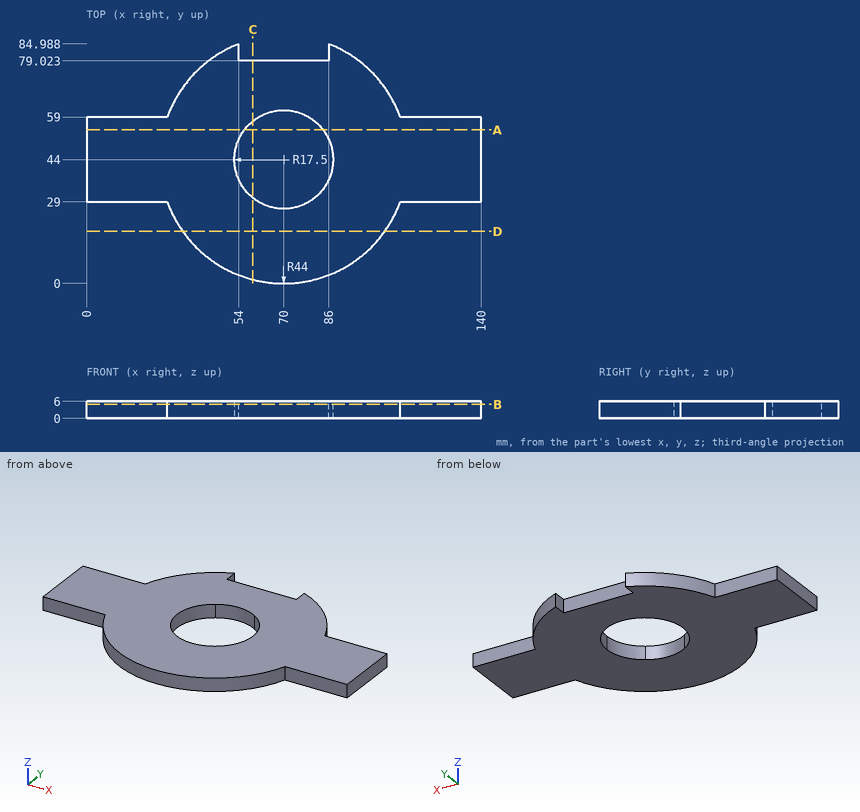
Job drawing, mm, ordinate dimensions from the low corner. One solid piece. Give positions to 0.01 mm unless a question says otherwise; leave off trailing zeros. Write each loop counter-clockwise with the first axis right and the second up, starting at its lowest first coordinate (ties: lowest second). Pieces come first, ordered by that corner, then holes. Notation, with made-up numbers: (-30.75, 5) - (22.25, 5) arc R33 ccw to (22.25, 34) - close; hole circle Ø11 at (76, 8). An arc over 180 degrees is marked (long way). Use one line per item in the form item = value. Start each with the question number.
1. Band-saw the part on C-C on x = 59. Write the cut outline in (y, z), plus the area to 3 significant figures.
2. Band-saw the part on A-A on y = 54.5. Write the cut outline in (x, z).
3. Band-saw the part on B-B on z = 5. Write the cut outline in (x, y), plus the area to 3 significant figures.
4. Drop flat-ended pins along their axis: pin 1 Ø1 at (x, z) = (31.5, 4.5) entering from +Y; pin 2 Ø3 at (x, z) = (14, 2) entering from -Y; pin 3 Ø3 at (y, z) = (20, 2) entering from +X. Give the stop position or say it passes through.
5. Probe line 1 (X direction, y = 45, z = 0.75); line 2 (Y direction, x = 71, z = 1.65); line 3 (Y direction, x = 16, z = 3.25). List the from-to ranges inside material, lowest first. Write a range as [from, to].
6. Band-saw the part on D-D on y = 18.5. Write the cut outline in (x, z), plus the area to 3 significant figures.
Conclusion:
q1.outline = (1.4, 0) - (30.39, 0) - (30.39, 6) - (1.4, 6) - close; (57.61, 0) - (79.02, 0) - (79.02, 6) - (57.61, 6) - close
q1.area = 302 mm²
q2.outline = (0, 0) - (56, 0) - (56, 6) - (0, 6) - close; (84, 0) - (140, 0) - (140, 6) - (84, 6) - close
q3.outline = (0, 29) - (28.64, 29) arc R44 ccw to (111.36, 29) - (140, 29) - (140, 59) - (111.36, 59) arc R44 ccw to (86, 84.99) - (86, 79.02) - (54, 79.02) - (54, 84.99) arc R44 ccw to (28.64, 59) - (0, 59) - close; hole circle Ø35 at (70, 44)
q3.area = 6,480 mm²
q4.pin_1 = 66.18
q4.pin_2 = 29
q4.pin_3 = 107.81
q5.line_1 = [0, 52.53], [87.47, 140]
q5.line_2 = [0.01, 26.53], [61.47, 79.02]
q5.line_3 = [29, 59]
q6.outline = (34.14, 0) - (105.86, 0) - (105.86, 6) - (34.14, 6) - close
q6.area = 430 mm²
